```python
from build123d import *

# Parameters (mm, degrees)
F0_R     = 266.5
F0_R_2   = 228.5
F1_DEPTH = 12.5
F3_D     = 11.50874


with BuildPart() as f1:
    # F0 (on Top) → F1 (new body)
    with BuildSketch(Plane.XY):
        Circle(F0_R)
        Circle(F0_R_2, mode=Mode.SUBTRACT)
    extrude(amount=F1_DEPTH)

    # F3 (through all)
    with Locations(Plane.XY.offset(12.5)):
        with Locations((-94.7141495104, 228.6601842965), (0, 247.5), (94.7141495104, 228.6601842965), (175.0089283437, 175.0089283437), (228.6601842965, 94.7141495104), (247.5, 0), (228.6601842965, -94.7141495104), (175.0089283437, -175.0089283437), (94.7141495104, -228.6601842965), (0, -247.5), (-94.7141495104, -228.6601842965), (-175.0089283437, -175.0089283437), (-228.6601842965, -94.7141495104), (-247.5, 0), (-228.6601842965, 94.7141495104), (-175.0089283437, 175.0089283437)):
            Hole(F3_D / 2)


solid = f1.part
```
Source: CAD feature listing. Evaluate the final solid. Frame: model axes, mm. Give positions to 0.01 mm unless a question says otherwise; leave off trailing zeros. Loops run counter-clockwise (first coordinate to the right, second up) from the corner with the lowest first, then second, coordinate; pieces in that order, holes last. Notation, with made-up numbers: (-39.5, 69) - (-23.5, 69) arc R19 cw to (-23.5, 88) - close; hole circle Ø6 at (24, 18.25). An arc over 180 degrees is marked (long way). Use CSV: the item, a comma, the result in double quotes. Start each with the question number.
1. Section A-A (y = -82). Output: boundary loops of the cut face in (x, z), then the cut area to 3 significant figures.
2. Pin query (flat end, axial travel): pin 1 (15 mm diameter, centred on x = -175.01, y = 175.01, fed in from +Z); pin 2 (1 mm diameter, centred on x = 170, z = 6.5, fed in from +Y); pin 3 (6 mm diameter, centred on y = -144.5, z = 10, fed in from -X); pin 4 (1 mm diameter, centred on x = 86.5, z = 7, fed in from -Y). Return the tip coordinate at first contact, or that it passes through.
3. Draft query along Y for faces 1 (the cylindrical face through (0.749, 253.205, 6.163)), 2 (the flat face through (78, -216, 0)), 3 (the cylindrical face through (-57.772, -260.163, 6.162)). Return one class per face: +Y half, -Y half, draft (parallel to the pull), parting line (faces both ways), or undercut.
4. Section C-C (z = 9.5). Count the separate pieces of the cut face and the enclosed holes in it, then the cut area to 3 significant figures.
5. Section B-B (x = 109.5). Output: boundary loops of the cut face in (y, z).
6. Ray query, L1, parallel to Y at x = 0, z = 4.5; L2, parallel to Y at x = 170, z = 6.75; L3, parallel to X at y = -31, z = 0.5. Return the intervals inside material, ascending.
Response:
1,outline,"(-253.57, 0) - (-213.28, 0) - (-213.28, 12.5) - (-253.57, 12.5) - close; (213.28, 0) - (253.57, 0) - (253.57, 12.5) - (213.28, 12.5) - close"
1,area,"1,010 mm²"
2,pin 1,"z = 12.5"
2,pin 2,"y = 205.65"
2,pin 3,"x = -225.83"
2,pin 4,"y = -252.24"
3,face 1,"undercut"
3,face 2,"draft"
3,face 3,"parting line"
4,separate pieces,"1"
4,enclosed holes,"17"
4,area,"57,400 mm²"
5,outline,"(-242.97, 0) - (-200.55, 0) - (-200.55, 12.5) - (-242.97, 12.5) - close; (200.55, 0) - (242.97, 0) - (242.97, 12.5) - (200.55, 12.5) - close"
6,L1,"-266.5 to -253.25, -241.75 to -228.5, 228.5 to 241.75, 253.25 to 266.5"
6,L2,"-205.24 to -177.84, -172.18 to -152.68, 152.68 to 172.18, 177.84 to 205.24"
6,L3,"-264.69 to -226.39, 226.39 to 264.69"
